Geometry: see drawing. Coordinates: mm, zero at the bounding-box minimum. Coordinates: 2 decimals unless noted, no trailing zeros. Loops run counter-clockwise (first coordinate to the right, second up) from the corner with the lowest first, then second, coordinate; pieces in that order, holes last. Notation, with made-up numbers: (-32.75, 3) -> (-24.75, 3) arc R23 cw to (-24.75, 37) -> close; hole circle Ø6 at (39, 86). An arc over 180 degrees is marked (long way). One line per item, written item: value. Start each with the question number.
Item 1: Section query B-B on y = 20. Return loops of the section in (x, z), then the cut area to 3 significant figures.
Item 2: Ray query, probe 1 along Y at (x, z) = (20, 0.8); probe 2 along X at (y, z) = (27, 0.35) (3 decimals); probe 3 along Y at (x, z) = (20.5, 0.5). Return the intervals inside material, ascending. Write a range as from..to.
Item 3: Section query A-A on x = 20. Return loops of the section in (y, z), then the cut area to 3 significant figures.
Item 4: Contact query for a flat-ended pin moving along its axis: pin 1 Ø7 at (x, y) = (20, 20) entering from -Z. Output: stop coordinate, or through.
Item 5: Section query C-C on z = 1. Return loops of the section in (x, y).
Item 6: Section query D-D on y = 28.1. Return loops of the section in (x, z), then the cut area to 3 significant figures.
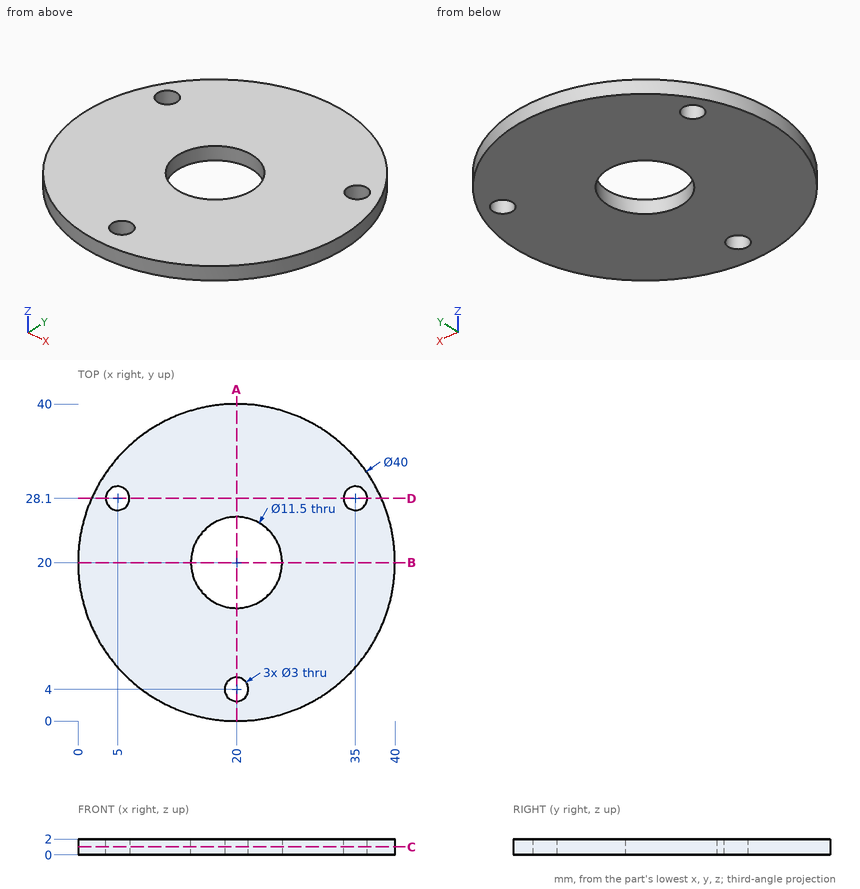
Reply:
1. outline: (0, 0) -> (14.25, 0) -> (14.25, 2) -> (0, 2) -> close; (25.75, 0) -> (40, 0) -> (40, 2) -> (25.75, 2) -> close
1. area: 57.0 mm²
2. probe 1: y = 0..2.5, 5.5..14.25, 25.75..40
2. probe 2: x = 1.265..3.98, 6.02..33.98, 36.02..38.735
2. probe 3: y = 0.01..2.59, 5.41..14.27, 25.73..39.99
3. outline: (0, 0) -> (2.5, 0) -> (2.5, 2) -> (0, 2) -> close; (5.5, 0) -> (14.25, 0) -> (14.25, 2) -> (5.5, 2) -> close; (25.75, 0) -> (40, 0) -> (40, 2) -> (25.75, 2) -> close
3. area: 51.0 mm²
4. pin 1: passes through
5. outline: circle Ø40 at (20, 20); hole circle Ø3 at (5, 28.1); hole circle Ø11.5 at (20, 20); hole circle Ø3 at (20, 4); hole circle Ø3 at (35, 28.1)
6. outline: (1.71, 0) -> (3.5, 0) -> (3.5, 2) -> (1.71, 2) -> close; (6.5, 0) -> (33.5, 0) -> (33.5, 2) -> (6.5, 2) -> close; (36.5, 0) -> (38.29, 0) -> (38.29, 2) -> (36.5, 2) -> close
6. area: 61.1 mm²
